Verification items for this drawing (mm, ordinates from the low corner). A direction names the side the tool comes from. Round coordinates to 2 decimals unless told otherwise and drop trailing zeros. Loops run counter-clockwise (first coordinate to the right, second up) from the corner with the lowest first, then second, coordinate; pieces in that order, holes last. Notation, with made-up numbers: (-15, 70.25) -> (18, 70.25) arc R30 ccw to (18, 108.25) -> close; hole circle Ø10 at (1, -30.75). An arc over 180 degrees is marked (long way). One line per item, written item: value. Start each with the question number.
1. Release check for a two-part mould opening along Y. For the marked faces 1, 2 and 3 record: +Y half, -Y half, draft (parallel to the pull), parting line (faces both ways), or undercut.
2. Cross-section at B-B on z = 10. Count the separate pieces of the cut face and the enclosed holes in it, then the cut area to 3 significant figures.
3. Cross-section at D-D on z = 15. Record the cut outline in (x, y).
4. Cross-section at C-C on y = 4.5. Record the cut outline in (x, z), then the cut area to 3 significant figures.
5. Set-up check for the marked faces 4, 5, 6 and 7: record each of +Z, -Z, +X, -X, +Y, -Y from which the full face is reachable in a straight line by a thin tool's end or side.
6. Cross-section at A-A on x = 39.5. Record the cut outline in (y, z), then the cut area to 3 significant figures.
7. Go/stop test with flat-tipped pins: pin 1 (2.5 mm diameter, centred on y = 83, z = 10, fed in from +X); pin 2 (5 mm diameter, centred on x = 39.5, y = 32, fed in from -Z); pin 3 (2.5 mm diameter, centred on x = 36.5, z = 16, fed in from -Y); pin 4 (4 mm diameter, centred on y = 62.5, z = 10.5, fed in from +X). Record where each tip stops, or that it passes through.
8. Material ranges on L1, parallel to Y at x = 48, z = 18.25; L2, parallel to Y at x = 39.5, z = 16.25; L3, parallel to Z at x = 1, y = 69, recorded low to high.
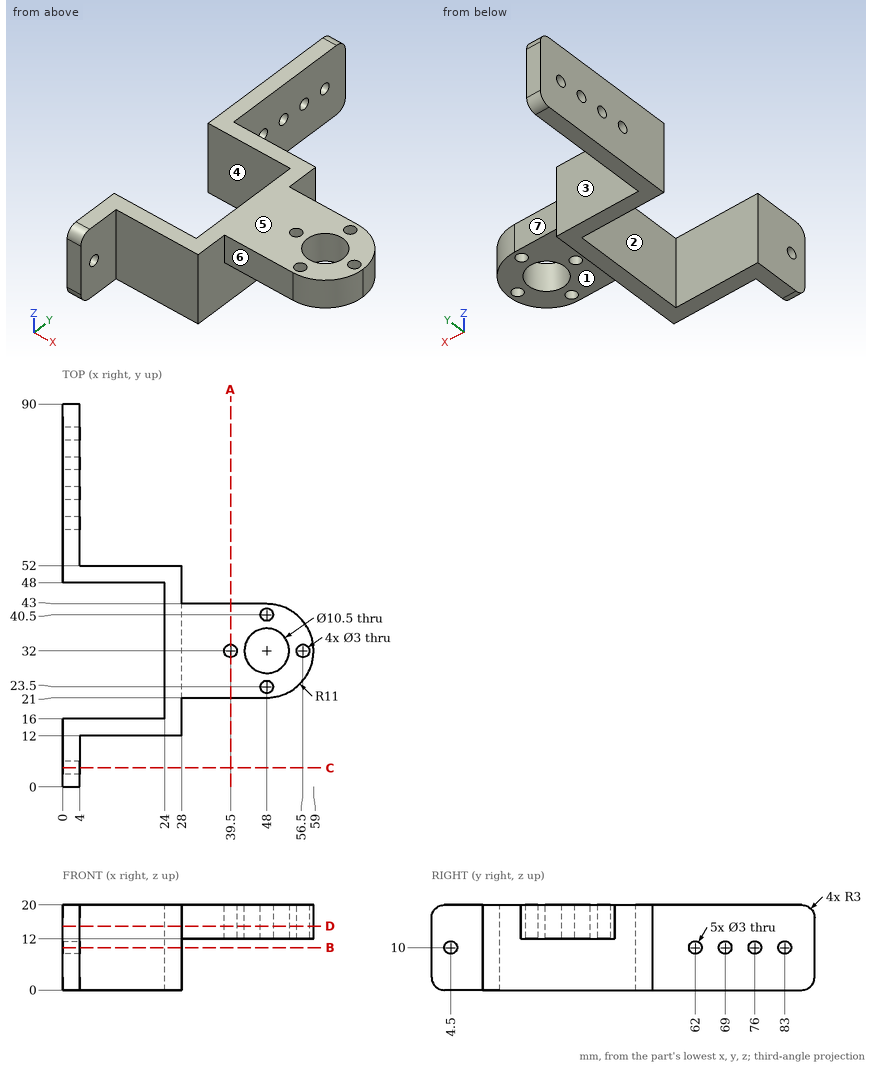
Taken from the geometry:
1. face 1: draft
1. face 2: undercut
1. face 3: +Y half
2. separate pieces: 6
2. enclosed holes: 0
2. area: 492 mm2
3. outline: (0, 0) -> (4, 0) -> (4, 12) -> (28, 12) -> (28, 21) -> (48, 21) arc R11 ccw to (48, 43) -> (28, 43) -> (28, 52) -> (4, 52) -> (4, 90) -> (0, 90) -> (0, 48) -> (24, 48) -> (24, 16) -> (0, 16) -> close; hole circle Ø3 at (39.5, 32); hole circle Ø10.5 at (48, 32); hole circle Ø3 at (48, 23.5); hole circle Ø3 at (48, 40.5); hole circle Ø3 at (56.5, 32)
4. outline: (0, 0) -> (4, 0) -> (4, 8.5) -> (0, 8.5) -> close; (0, 11.5) -> (4, 11.5) -> (4, 20) -> (0, 20) -> close
4. area: 68.0 mm2
5. face 4: +Z, -Z, -X
5. face 5: +Z, +X, -X, +Y, -Y
5. face 6: +Z, -Z, +X, -Y
5. face 7: +Z, -Z, +X, +Y
6. outline: (21, 12) -> (30.5, 12) -> (30.5, 20) -> (21, 20) -> close; (33.5, 12) -> (43, 12) -> (43, 20) -> (33.5, 20) -> close
6. area: 152 mm2
7. pin 1: passes through
7. pin 2: stops at z = 12
7. pin 3: stops at y = 21
7. pin 4: stops at x = 4
8. L1: y = 21 to 22, 25 to 26.75, 37.25 to 39, 42 to 43
8. L2: y = 21 to 30.5, 33.5 to 43
8. L3: z = 0 to 8.5, 11.5 to 20
